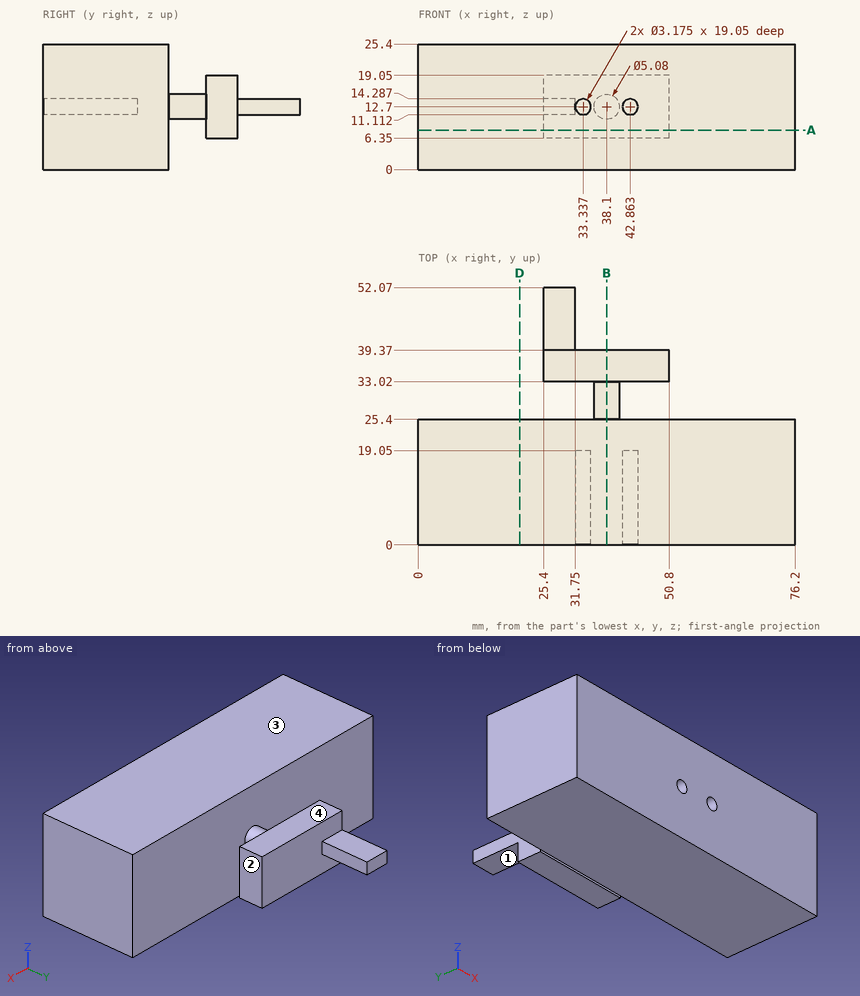
Geometry: see drawing. Coordinates: mm, zero at the bounding-box minimum. A direction names the side the tool comes from. Give positions to 0.01 mm unless a question says otherwise; leave off trailing zeros. Loops run counter-clockwise (first coordinate to the right, second up) from the corner with the lowest first, then second, coordinate; pieces in that order, holes last. Notation, with made-up numbers: (81.25, -40) - (124.25, -40) arc R7 ccw to (124.25, -32) - close; hole circle Ø7 at (-9, -1.5). An arc over 180 degrees is marked (long way). Use CSV: the item, a comma, the result in double quotes. Start each with the question number.
Item 1: Section B-B on x = 38.1. Return loops of the section in (y, z).
Item 2: Contact query for flat-ended pins moving along their axis: P1, Ø1.9, axis at x = 42, y = 37, coming from the +Z side; P2, Ø5, axis at x = 58.5, z = 4, coming from the +Y side; P3, Ø1.9, axis at x = 28, y = 44.5, coming from the +Z side. Output: stop coordinate, or through.
Item 3: Section A-A on z = 8. Return loops of the section in (x, y).
Item 4: Reachability of the marked faces 1, 2, 3 and 4 from +Z, -Z, +X, -X, +Y, -Y: full face, straight path, thin tool, end or side. Return the list, or none.
Item 5: Line query: line 1 (Y direction, x = 9, z = 22.5); line 2 (X direction, y = 36, z = 8.75); line 3 (Y direction, x = 33, z = 10.5). Output: solid intervals per line, ascending.
Item 6: Section D-D on x = 20.5. Return loops of the section in (y, z), then the cut area to 3 significant figures.
Ans:
1,outline,"(0, 0) - (25.4, 0) - (25.4, 10.16) - (33.02, 10.16) - (33.02, 6.35) - (39.37, 6.35) - (39.37, 19.05) - (33.02, 19.05) - (33.02, 15.24) - (25.4, 15.24) - (25.4, 25.4) - (0, 25.4) - close"
2,P1,"stops at z = 19.05"
2,P2,"stops at y = 25.4"
2,P3,"stops at z = 14.29"
3,outline,"(0, 0) - (76.2, 0) - (76.2, 25.4) - (0, 25.4) - close; (25.4, 33.02) - (50.8, 33.02) - (50.8, 39.37) - (25.4, 39.37) - close"
4,face 1,"-Z, +X, -X, +Y"
4,face 2,"+Z, -Z, +X, +Y"
4,face 3,"+Z, +X, -X, +Y, -Y"
4,face 4,"+Z, +X, -X, +Y"
5,line 1,"y = 0 to 25.4"
5,line 2,"x = 25.4 to 50.8"
5,line 3,"y = 0 to 25.4, 33.02 to 39.37"
6,outline,"(0, 0) - (25.4, 0) - (25.4, 25.4) - (0, 25.4) - close"
6,area,"645 mm2"
